from build123d import *

# Parameters (mm, degrees)
SKETCH_1_W                    = 4
SKETCH_1_H                    = 55
REVOLVE_1_ANGLE               = 180
SKETCH_2_W                    = 4
SKETCH_2_H                    = 110
EXTRUDE_1_DEPTH               = 150
EXTRUDE_2_DEPTH               = 38
CUT_EXTRUDE_1_DEPTH           = 40
SKETCH_5_W                    = 36.5
SKETCH_5_H                    = 54.5
EXTRUDE_3_DEPTH               = 17
SKETCH_6_W                    = 31.5
SKETCH_6_H                    = 49.5
CUT_EXTRUDE_2_DEPTH           = 17
HOLE_WIZARD_20_0_20_1_D       = 20
HOLE_WIZARD_20_0_20_1_DEPTH   = 2
HOLE_WIZARD_10_0_10_1_D       = 10
HOLE_WIZARD_10_0_10_1_DEPTH   = 2
HOLE_WIZARD_2_5_2_5_1_D       = 2.5
HOLE_WIZARD_2_5_2_5_1_DEPTH   = 4
HOLE_WIZARD_2_05_2_05_1_D     = 2.05
HOLE_WIZARD_2_05_2_05_1_DEPTH = 2.5
HOLE_WIZARD_2_05_2_05_2_D     = 2.05
HOLE_WIZARD_2_05_2_05_2_DEPTH = 2.5
HOLE_WIZARD_2_05_2_05_3_D     = 2.05
HOLE_WIZARD_2_05_2_05_3_DEPTH = 2.5
HOLE_WIZARD_2_05_2_05_4_D     = 2.05
HOLE_WIZARD_2_05_2_05_4_DEPTH = 2.5
FILLET_1_R                    = 4


with BuildPart() as part:
    # 스케치1 → 회전1 (revolve)
    with BuildSketch(Plane.XZ.offset(-35.25)):
        with Locations((-21, -41.75)):
            Rectangle(SKETCH_1_W, SKETCH_1_H)
    revolve(axis=Axis((-18.999896922, 35.25, -14.25), (1, 0, 0)), revolution_arc=REVOLVE_1_ANGLE)

    # 스케치2 → 보스-돌출1 (add)
    with BuildSketch(Plane.XZ.offset(-35.25)):
        with Locations((-21, -14.25)):
            Rectangle(SKETCH_2_W, SKETCH_2_H)
    extrude(amount=EXTRUDE_1_DEPTH)

    # 스케치3 → 보스-돌출2 (add)
    with BuildSketch(Plane(origin=(-19, 0, 0), x_dir=(0, 0, -1), z_dir=(1, 0, 0))):
        with BuildLine():
            Line((-25.75, -114.75), (-25.75, 35.25))
            ThreePointArc((-25.75, 35.25), (14.25, 75.25), (54.25, 35.25))
            Line((54.25, 35.25), (54.25, -114.75))
            Line((54.25, -114.75), (-25.75, -114.75))
        make_face()
    extrude(amount=EXTRUDE_2_DEPTH)

    # 스케치4 → 컷-돌출1 (cut)
    with BuildSketch(Plane.ZY.offset(23)):
        with BuildLine():
            Line((-50.25, -110.75), (21.75, -110.75))
            Line((21.75, -110.75), (21.75, 35.25))
            ThreePointArc((21.75, 35.25), (-14.25, 71.25), (-50.25, 35.25))
            Line((-50.25, 35.25), (-50.25, -110.75))
        make_face()
    extrude(amount=-CUT_EXTRUDE_1_DEPTH, mode=Mode.SUBTRACT)

    # 스케치5 → 보스-돌출3 (add)
    with BuildSketch(Plane.ZY.offset(-17)):
        with Locations((-14.25, 23.25)):
            Rectangle(SKETCH_5_W, SKETCH_5_H)
    extrude(amount=EXTRUDE_3_DEPTH)

    # 스케치6 → 컷-돌출2 (cut)
    with BuildSketch(Plane.ZY):
        with Locations((-14.25, 23.25)):
            Rectangle(SKETCH_6_W, SKETCH_6_H)
    extrude(amount=-CUT_EXTRUDE_2_DEPTH, mode=Mode.SUBTRACT)

    # Ø20.0 (20) 지름 구멍1
    with Locations(Plane.ZY.offset(-17)):
        with Locations((-14.25, 35.25)):
            Hole(HOLE_WIZARD_20_0_20_1_D / 2, depth=HOLE_WIZARD_20_0_20_1_DEPTH)

    # Ø10.0 (10) 지름 구멍1
    with Locations(Plane.ZY.offset(-17)):
        with Locations((-14.25, -76.75)):
            Hole(HOLE_WIZARD_10_0_10_1_D / 2, depth=HOLE_WIZARD_10_0_10_1_DEPTH)

    # Ø2.5 (2.5) 지름 구멍1
    with Locations(Plane(origin=(-19, 0, 0), x_dir=(0, 0, -1), z_dir=(1, 0, 0))):
        with Locations((-34.75, -104.75), (63.25, -104.75), (63.25, -39.75), (63.25, 35.25), (-34.75, 35.25), (-34.75, -39.75), (14.25, 84.25)):
            Hole(HOLE_WIZARD_2_5_2_5_1_D / 2, depth=HOLE_WIZARD_2_5_2_5_1_DEPTH)

    # Ø2.05 (2.05) 지름 구멍1
    with Locations(Plane(origin=(0, -1.5, 0), x_dir=(1, 0, 0), z_dir=(0, 1, 0))):
        with Locations((6, 6.25), (6, 22.25)):
            Hole(HOLE_WIZARD_2_05_2_05_1_D / 2, depth=HOLE_WIZARD_2_05_2_05_1_DEPTH)

    # Ø2.05 (2.05) 지름 구멍2
    with Locations(Plane(origin=(0, 0, 1.5), x_dir=(-1, 0, 0), z_dir=(0, 0, -1))):
        with Locations((-6, 27.25), (-6, 3.25)):
            Hole(HOLE_WIZARD_2_05_2_05_2_D / 2, depth=HOLE_WIZARD_2_05_2_05_2_DEPTH)

    # Ø2.05 (2.05) 지름 구멍3
    with Locations(Plane(origin=(0, 48, 0), x_dir=(-1, 0, 0), z_dir=(0, -1, 0))):
        with Locations((-6, 6.25), (-6, 22.25)):
            Hole(HOLE_WIZARD_2_05_2_05_3_D / 2, depth=HOLE_WIZARD_2_05_2_05_3_DEPTH)

    # Ø2.05 (2.05) 지름 구멍4
    with Locations(Plane.XY.offset(-30)):
        with Locations((6, 27.25), (6, 3.25)):
            Hole(HOLE_WIZARD_2_05_2_05_4_D / 2, depth=HOLE_WIZARD_2_05_2_05_4_DEPTH)

    # 필렛1
    fillet_1_edges = [part.edges().sort_by_distance(p)[0] for p in [
        (-19, -39.75, -54.25),
        (-19, 75.25, -14.25),
        (-19, -39.75, 25.75),
    ]]
    fillet(fillet_1_edges, radius=FILLET_1_R)


solid = part.part
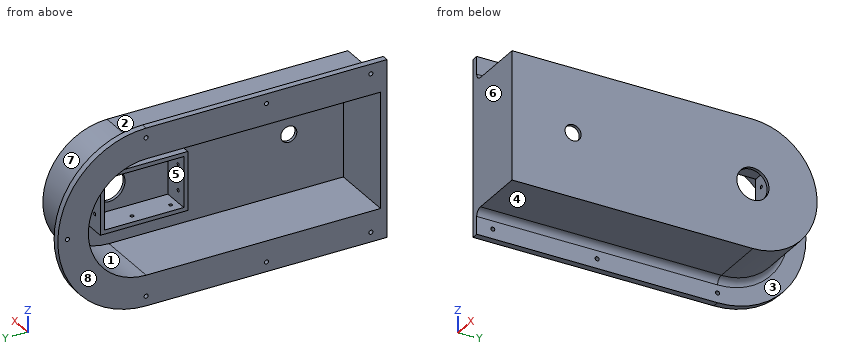
For this review, take the finished solid that the model builds, in its own axes (mm). Face numbers are marked on the shaded views. A direction names the side the tool comes from. Coordinates: 2 decimals unless noted, no trailing zeros. Order: outer loops, then holes, each group sorted by start corner. A loop starts at its lowest first (then second) coordinate and runs counter-clockwise, first axis right, second up. Notation, with made-up numbers: (32.5, -27) -> (68.5, -27) arc R24 ccw to (68.5, -6) -> close; hole circle Ø5 at (78, 41.25). An arc over 180 degrees is marked (long way). Return JSON: item names as keys, results as strings.
1. The part is to be moulded in two halves that separate along Z. For the marked faces 1, 2 and 3, say which applies: +Z half, -Z half, draft (parallel to the pull), parting line (faces both ways), or undercut.
Answer block:
{"face 1": "undercut", "face 2": "+Z half", "face 3": "draft"}
2. We need section B-B on y = -14. Write out the cut boundary in (x, z), and give its area (3 significant figures).
Answer block:
{"outline": "(-23, -69.25) -> (-19, -69.25) -> (-19, -58.25) arc R4 cw to (-15, -54.25) -> (19, -54.25) -> (19, 25.75) -> (-15, 25.75) arc R4 cw to (-19, 29.75) -> (-19, 40.75) -> (-23, 40.75) -> (-23, 21.75) -> (17, 21.75) -> (17, -50.25) -> (-23, -50.25) -> close", "area": "607 mm²"}
3. For line 1 (Z direction, x = -6, y = -6); line 2 (Z direction, x = 6, y = 49.65) (3 decimals); line 3 (Z direction, x = -21, y = 35), list the stretches that pass through material, from the lowest coordinate up. Write a range as from..to.
Answer block:
{"line 1": "-54.25..-50.25, 21.75..25.75", "line 2": "-51.568..-47.245, -32.5..-23.275, -21.225..-7.275, -5.225..4, 18.745..23.068", "line 3": "-69.25..-64.47, -62.03..-50.25, 21.75..33.53, 35.97..40.75"}
4. Machinability: for the marked faces 4, 5, 6, 7 and 8, which of the approach directions +Z, -Z, +X, -X, +Y, -Y give a long, thin tool a straight path to every point of the face, cutting with its end or side? Answer none if there is none.
Answer block:
{"face 4": "-Z, +X, +Y, -Y", "face 5": "-X", "face 6": "+Z, -Z, +X, -X, -Y", "face 7": "+X, +Y", "face 8": "+Z, -Z, -X, +Y, -Y"}
5. We need section A-A on x = -9. Write out the cut boundary in (y, z), and give its area (3 significant figures).
Answer block:
{"outline": "(-114.75, -54.25) -> (35.25, -54.25) arc R40 ccw to (35.25, 25.75) -> (-114.75, 25.75) -> close; hole (-110.75, -50.25) -> (35.25, -50.25) arc R36 ccw to (35.25, 21.75) -> (-110.75, 21.75) -> close", "area": "1,970 mm²"}
6. For pin 1 Ø1 at (y, z) = (-30.5, 20) entering from -X; pin 2 Ø1 at (x, y) = (3.5, 16) entering from +Z; pin 3 Ø3 at (x, y) = (12.5, 65) entering from -Z, all flat-tipped, find the tip position at first contact; note any pin that passes through.
Answer block:
{"pin 1": "x = 17", "pin 2": "z = 25.75", "pin 3": "z = -42.57"}
